```python
from build123d import *

# Parameters (mm, degrees)
SKETCH_4_W        = 44
SKETCH_4_H        = 20
EXTRUDE_282_DEPTH = 1.5
SKETCH_5_W        = 3
SKETCH_5_H        = 20
EXTRUDE_1_DEPTH   = 5.5
EXTRUDE_START     = 4
SKETCH_6_W        = 12
SKETCH_6_H        = 20
EXTRUDE_1_2_DEPTH = 1.5
SKETCH_7_W        = 1.5
SKETCH_7_H        = 20
EXTRUDE_1_3_DEPTH = 48
SKETCH_8_W        = 3
SKETCH_8_H        = 20
EXTRUDE_1_4_DEPTH = 5.5
SKETCH_9_W        = 12
SKETCH_9_H        = 20
EXTRUDE_1_5_DEPTH = 1.5
SKETCH_10_W       = 1.5
SKETCH_10_H       = 20
EXTRUDE_1_6_DEPTH = 48
EXTRUDE_START_2   = 52
SKETCH_11_W       = 66
SKETCH_11_H       = 20
EXTRUDE_763_DEPTH = 1.5


with BuildPart() as part:
    # 草图4 → Extrude 282 (new body)
    with BuildSketch(Plane.XY):
        Rectangle(SKETCH_4_W, SKETCH_4_H)
    extrude(amount=EXTRUDE_282_DEPTH)

    # 草图5 → Extrude 1 (add)
    with BuildSketch(Plane.XY):
        with Locations((-21.5, 0)):
            Rectangle(SKETCH_5_W, SKETCH_5_H)
    extrude(amount=EXTRUDE_1_DEPTH)

    # 草图6 → Extrude 1 2 (add)
    with BuildSketch(Plane.XY.offset(EXTRUDE_START)):
        with Locations((-27, 0)):
            Rectangle(SKETCH_6_W, SKETCH_6_H)
    extrude(amount=EXTRUDE_1_2_DEPTH)

    # 草图7 → Extrude 1 3 (add)
    with BuildSketch(Plane.XY.offset(EXTRUDE_START)):
        with Locations((-32.25, 0)):
            Rectangle(SKETCH_7_W, SKETCH_7_H)
    extrude(amount=EXTRUDE_1_3_DEPTH)

    # 草图8 → Extrude 1 4 (add)
    with BuildSketch(Plane.XY):
        with Locations((21.5, 0)):
            Rectangle(SKETCH_8_W, SKETCH_8_H)
    extrude(amount=EXTRUDE_1_4_DEPTH)

    # 草图9 → Extrude 1 5 (add)
    with BuildSketch(Plane.XY.offset(EXTRUDE_START)):
        with Locations((27, 0)):
            Rectangle(SKETCH_9_W, SKETCH_9_H)
    extrude(amount=EXTRUDE_1_5_DEPTH)

    # 草图10 → Extrude 1 6 (add)
    with BuildSketch(Plane.XY.offset(EXTRUDE_START)):
        with Locations((32.25, 0)):
            Rectangle(SKETCH_10_W, SKETCH_10_H)
    extrude(amount=EXTRUDE_1_6_DEPTH)

    # 草图11 → Extrude 763 (add)
    with BuildSketch(Plane.XY.offset(EXTRUDE_START_2)):
        Rectangle(SKETCH_11_W, SKETCH_11_H)
    extrude(amount=EXTRUDE_763_DEPTH)


solid = part.part
```
The model under review builds one solid part; all positions refer to its coordinate system, in mm. A direction names the side the tool comes from. Round coordinates to 2 decimals unless told otherwise and drop trailing zeros. Order: outer loops, then holes, each group sorted by start corner. A loop starts at its lowest first (then second) coordinate and runs counter-clockwise, first axis right, second up.
Item 1: Add section A-A, the plane z = 30. State the section outline as (x, y) points, and give its area (3 significant figures).
Working result:
outline: (-33, -10) - (-31.5, -10) - (-31.5, 10) - (-33, 10) - close; (31.5, -10) - (33, -10) - (33, 10) - (31.5, 10) - close
area: 60.0 mm2
Item 2: For pin 1 (12 mm diameter, centred on x = -19.5, z = 16, fed in from -Y); pin 2 (5 mm diameter, centred on x = 28, y = 0, fed in from -Z); pin 3 (2 mm diameter, centred on x = 14, y = 5, fed in from -Z), all flat-tipped, find the tip position at first contact; note any pin that passes through.
Working result:
pin 1: passes through
pin 2: stops at z = 4
pin 3: stops at z = 0
Item 3: Add section B-B, the plane x = 21. State the section outline as (y, z) points.
Working result:
outline: (-10, 0) - (10, 0) - (10, 5.5) - (-10, 5.5) - close; (-10, 52) - (10, 52) - (10, 53.5) - (-10, 53.5) - close
Item 4: Draft analysis for pull direction Z (two halves, no side actions). For faces 1 (the flat face through (0, 0, 53.5)), 2 (the flat face through (-2.6, -10, 52.4)), 3 (the flat face through (26, 0, 5.5)), state which applies: released by +Z, released by -Z, zero draft, split by the parting line, or undercut.
Working result:
face 1: released by +Z
face 2: zero draft
face 3: undercut
Item 5: To check wall thickness, follow probe 1 along Z at (x, y) = (14.5, 9.25); probe 2 along X at (y, z) = (1.25, 16.5); probe 3 along Z at (x, y) = (27.5, 6.25). State the ranges of each line that lie inside material, in increasing order.
Working result:
probe 1: z = 0 to 1.5, 52 to 53.5
probe 2: x = -33 to -31.5, 31.5 to 33
probe 3: z = 4 to 5.5, 52 to 53.5
Item 6: Add section C-C, the plane y = 0.5. State the section outline as (x, z) points.
Working result:
outline: (-33, 4) - (-23, 4) - (-23, 0) - (23, 0) - (23, 4) - (33, 4) - (33, 53.5) - (-33, 53.5) - close; hole (-31.5, 5.5) - (-20, 5.5) - (-20, 1.5) - (20, 1.5) - (20, 5.5) - (31.5, 5.5) - (31.5, 52) - (-31.5, 52) - close
Item 7: Machinability: for faces 4 (the flat face through (23, 0, 2)), 5 (the flat face through (-26, 0, 5.5)), 6 (the flat face through (-33, 0, 28)), 7 (the flat face through (-23, 0, 2)), 8 (the flat face through (33, 0, 28)), which of the approach directions +Z, -Z, +X, -X, +Y, -Y give a long, thin tool a straight path to every point of the face, cutting with its end or side? Answer none if there is none.
Working result:
face 4: -Z, +X, +Y, -Y
face 5: +Y, -Y
face 6: +Z, -Z, -X, +Y, -Y
face 7: -Z, -X, +Y, -Y
face 8: +Z, -Z, +X, +Y, -Y
